Design review of the part built by this model. Coordinates are the model's own, in mm. A direction names the side the tool comes from. Give positions to 0.01 mm unless a question says otherwise; leave off trailing zeros. Loops run counter-clockwise (first coordinate to the right, second up) from the corner with the lowest first, then second, coordinate; pieces in that order, holes last. Notation, with made-up numbers: (61.5, 63) -> (113.5, 63) arc R36 cw to (113.5, 102) -> close; hole circle Ø9 at (-7.75, 11.5). An arc over 180 degrees is marked (long way). Answer in a Markdown table with one row per item. Add a question column.
(1) For line 1 (X direction, y = 0.65, z = -9); line 2 (X direction, y = 0.9, z = -4); line 3 (X direction, y = 1.35, z = -3), list the stretches that pass through material, from the lowest coordinate up.
(2) For pin 1 (0.5 mm diameter, centred on y = 1, z = -8.5, fed in from -X), flat-tipped, find the tip position at first contact; note if it passes through.
(3) Draft analysis for pull direction Z (two halves, no side actions). For faces 4 (the flat face through (-9, 1, -12)), 5 (the cylindrical face through (-3.4, 0.8, 7.8)), 6 (the flat face through (-15, 1.6, 14)), state which applies: +Z half, -Z half, draft (parallel to the pull), parting line (faces both ways), or undercut.
(4) Consider section D-D on y = 0.45. Write out the cut boundary in (x, z), then the cut area to 3 significant figures.
(5) Consider section A-A on z = -9. Write out the cut boundary in (x, y).
(6) Consider section B-B on x = -2.5. Write out the cut boundary in (y, z), then the cut area to 3 significant figures.
(7) Consider section C-C on z = 9. Write out the cut boundary in (x, y), then the cut area to 3 significant figures.
(8) For faces 1 (the flat face through (-17, 1, -5)), 2 (the flat face through (-9, 1.4, 0)), 3 (the flat face through (-8, 1.6, -9)), list the 3-axis set-ups (+Z, -Z, +X, -X, +Y, -Y) from which the entire face can be reached by the end or side of a thin tool; tool diameter is ignored.
from build123d import *

# Parameters (mm, degrees)
EXTRUSION1_DEPTH        = 1.6
ESQUISSE2_R             = 0.9
ENL_V_MAT_EXTRU_1_DEPTH = 37.654604076
ENL_V_MAT_EXTRU_2_DEPTH = 0.2
ESQUISSE4_R             = 1.5
ENL_V_MAT_EXTRU_3_DEPTH = 37.654604076


with BuildPart() as part:
    # Esquisse1 → Extrusion1 (new body)
    with BuildSketch(Plane(origin=(0, 0, 0), x_dir=(1, 0, 0), z_dir=(0, 1, 0))):
        Polygon((-17, 12), (0, 12), (0, -21), (-30, -21), (-30, -15), (-17, -2), align=None)
    extrude(amount=EXTRUSION1_DEPTH)

    # Esquisse2 → Enlèv. mat.-Extru.1 (cut, through all)
    with BuildSketch(Plane(origin=(0, 1.6, 0), x_dir=(1, 0, 0), z_dir=(0, 1, 0))):
        with Locations(Location((-12.719630786, 3.685060513, 0), (0, 0, 270))):
            Circle(ESQUISSE2_R)
        with Locations(Location((-10.215884924, 3.201576633, 0), (0, 0, 270))):
            Circle(ESQUISSE2_R)
    extrude(amount=-ENL_V_MAT_EXTRU_1_DEPTH, mode=Mode.SUBTRACT)

    # Esquisse3 → Enlèv. mat.-Extru.2 (cut)
    with BuildSketch(Plane(origin=(0, 1.6, 0), x_dir=(1, 0, 0), z_dir=(0, 1, 0))):
        Polygon((-17, 7.782827883), (-17, -2), (-17.470712916, -2.470712916), (0, -7.368289602), (0, 3.017206465), align=None)
    extrude(amount=-ENL_V_MAT_EXTRU_2_DEPTH, mode=Mode.SUBTRACT)

    # Esquisse4 → Enlèv. mat.-Extru.3 (cut, through all)
    with BuildSketch(Plane(origin=(0, 1.6, 0), x_dir=(1, 0, 0), z_dir=(0, 1, 0))):
        with Locations(Location((-2.5, 9, 0), (0, 0, 270))):
            Circle(ESQUISSE4_R)
        with Locations(Location((-2.5, -9, 0), (0, 0, 270))):
            Circle(ESQUISSE4_R)
    extrude(amount=-ENL_V_MAT_EXTRU_3_DEPTH, mode=Mode.SUBTRACT)


solid = part.part
Values follow:
| question | item | result |
|---|---|---|
| 1 | line 1 | -17 to -4, -1 to 0 |
| 1 | line 2 | -17 to -13.56, -11.88 to -10.63, -9.8 to 0 |
| 1 | line 3 | -17 to -13.3, -12.14 to -11.09, -9.34 to 0 |
| 2 | pin 1 | x = -17 |
| 3 | face 4 | -Z half |
| 3 | face 5 | undercut |
| 3 | face 6 | draft |
| 4 | outline | (-30, 15) -> (-17, 2) -> (-17, -12) -> (0, -12) -> (0, 21) -> (-30, 21) -> close; hole circle Ø1.8 at (-12.72, -3.69); hole circle Ø1.8 at (-10.22, -3.2); hole circle Ø3 at (-2.5, -9); hole circle Ø3 at (-2.5, 9) |
| 4 | area | 704 mm2 |
| 5 | outline | (-17, 0) -> (-4, 0) -> (-4, 1.6) -> (-17, 1.6) -> close; (-1, 0) -> (0, 0) -> (0, 1.6) -> (-1, 1.6) -> close |
| 6 | outline | (0, -12) -> (1.6, -12) -> (1.6, -10.5) -> (0, -10.5) -> close; (0, -7.5) -> (1.6, -7.5) -> (1.6, -3.72) -> (1.4, -3.72) -> (1.4, 6.67) -> (1.6, 6.67) -> (1.6, 7.5) -> (0, 7.5) -> close; (0, 10.5) -> (1.6, 10.5) -> (1.6, 21) -> (0, 21) -> close |
| 6 | area | 41.1 mm2 |
| 7 | outline | (-24, 0) -> (-4, 0) -> (-4, 1.6) -> (-24, 1.6) -> close; (-1, 0) -> (0, 0) -> (0, 1.6) -> (-1, 1.6) -> close |
| 7 | area | 33.6 mm2 |
| 8 | face 1 | -Z, -X, +Y, -Y |
| 8 | face 2 | +Y |
| 8 | face 3 | +Z, -Z, +X, -X, +Y |
